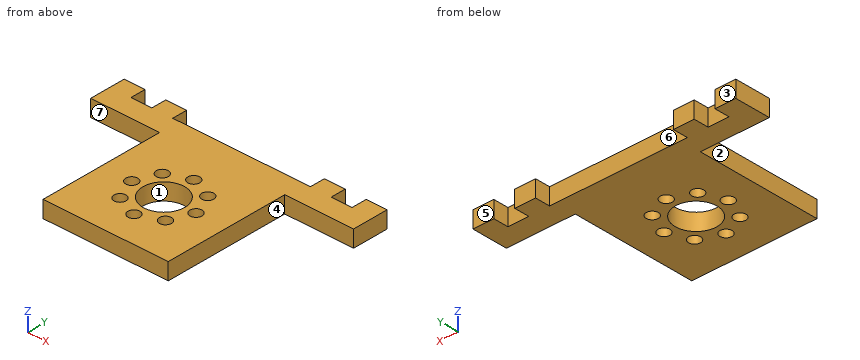
from build123d import *

# Parameters (mm, degrees)
BOSS_EXTRUDE1_DEPTH = 5.08
SKETCH3_W           = 6.35
SKETCH3_H           = 4.572
BOSS_EXTRUDE2_DEPTH = 5.08
SKETCH4_R           = 6.35
SKETCH4_R_2         = 1.8288
CUT_EXTRUDE1_DEPTH  = 5.08
SKETCH5_W           = 29.19984
SKETCH5_H           = 4.572
CUT_EXTRUDE2_DEPTH  = 5.08


with BuildPart() as part:
    # Sketch1 → Boss-Extrude1 (new body)
    with BuildSketch(Plane.XY):
        Polygon((-22.91953125, 7.590234375), (-22.91953125, 1.240234375), (-1.96961125, 1.240234375), (-1.96961125, -36.859765625), (36.13038875, -36.859765625), (36.13038875, 1.240234375), (57.08030875, 1.240234375), (57.08030875, 7.590234375), align=None)
    extrude(amount=BOSS_EXTRUDE1_DEPTH)

    # Sketch3 → Boss-Extrude2 (add)
    with BuildSketch(Plane(origin=(0, 0, 0), x_dir=(-1, 0, 0), z_dir=(0, 0, -1))):
        with Locations((19.74453125, 9.876234375)):
            Rectangle(SKETCH3_W, SKETCH3_H)
        with Locations((7.04453125, 9.876234375)):
            Rectangle(SKETCH3_W, SKETCH3_H)
        with Locations((-5.65546875, 9.876234375)):
            Rectangle(SKETCH3_W, SKETCH3_H)
        with Locations((-28.50530875, 9.876234375)):
            Rectangle(SKETCH3_W, SKETCH3_H)
        with Locations((-41.20530875, 9.876234375)):
            Rectangle(SKETCH3_W, SKETCH3_H)
        with Locations((-53.90530875, 9.876234375)):
            Rectangle(SKETCH3_W, SKETCH3_H)
    extrude(amount=-BOSS_EXTRUDE2_DEPTH)

    # Sketch4 → Cut-Extrude1 (cut)
    with BuildSketch(Plane.XY.offset(5.08)):
        with Locations((17.08038875, -17.809765625)):
            Circle(SKETCH4_R)
        with Locations((7.30138875, -17.809765625)):
            Circle(SKETCH4_R_2)
        with Locations((10.165591537, -10.894968412)):
            Circle(SKETCH4_R_2)
        with Locations((17.08038875, -8.030765625)):
            Circle(SKETCH4_R_2)
        with Locations((23.995185963, -10.894968412)):
            Circle(SKETCH4_R_2)
        with Locations((26.85938875, -17.809765625)):
            Circle(SKETCH4_R_2)
        with Locations((23.995185963, -24.724562838)):
            Circle(SKETCH4_R_2)
        with Locations((17.08038875, -27.588765625)):
            Circle(SKETCH4_R_2)
        with Locations((10.165591537, -24.724562838)):
            Circle(SKETCH4_R_2)
    extrude(amount=-CUT_EXTRUDE1_DEPTH, mode=Mode.SUBTRACT)

    # Sketch5 → Cut-Extrude2 (cut)
    with BuildSketch(Plane.XY.offset(5.08)):
        with Locations((17.08038875, 9.876234375)):
            Rectangle(SKETCH5_W, SKETCH5_H)
    extrude(amount=-CUT_EXTRUDE2_DEPTH, mode=Mode.SUBTRACT)


solid = part.part
Read the model definition and answer for the solid it produces. Units are mm, in the model's axes. Face numbers are marked on the shaded views. A direction names the side the tool comes from. Give positions to 0.01 mm unless a question says otherwise; leave off trailing zeros. Write each loop counter-clockwise with the first axis right and the second up, starting at its lowest first coordinate (ties: lowest second). Pieces come first, ordered by that corner, then holes. Notation, with made-up numbers: (77.5, 85.25) - (126.5, 85.25) arc R26 cw to (126.5, 115.25) - close; hole circle Ø5 at (86, 62). An arc over 180 degrees is marked (long way). Use CSV: the item, a comma, the result in double quotes. Start each with the question number.
(1) Given P1, Ø1.5, axis at x = -7.5, z = 1.5, coming from the -Y side; P2, Ø2, axis at y = -3.5, z = 3.5, coming from the +X side; P3, Ø2.5, axis at x = 48, z = 1.5, coming from the +Y side, each flat-ended and moving along its own axis, determine where each tip first touches the part or whether it passes through.
(2) Find section C-C (z = 1). Count the separate pieces of the cut face and the enclosed holes in it, plus the area to 4 significant figures.
(3) Find section A-A (x = 18). Give the vertices of the cut face in (y, z).
(4) For the marked faces 4, 5, 6 and 7, determine the directions among +Z, -Z, +X, -X, +Y, -Y from which every point of the face is accessible in a straight line to the end or side of a thin tool.
(5) Find section D-D (x = 47). Give the vertices of the cut face in (y, z), plus the area to 3 significant figures.
(6) Find section B-B (y = -22). Give the vertices of the cut face in (x, z).
(7) Consider line 1 along X through (y, z) = (-27.5, 3.9); line 2 along X through (y, z) = (-14, 3.85); line 3 along Y through (x, z) = (-10, 2.1). Determine where each line is inside the solid, lowest interval first.
(8) Determine the mould class of the marked faces 1, 2 and 3 for opening direction Y: +Y half, -Y half, draft (parallel to the pull), parting line (faces both ways), or undercut.
Findings below:
1,P1,"y = 1.24"
1,P2,"x = 36.13"
1,P3,"y = 7.59"
2,separate pieces,"1"
2,enclosed holes,"9"
2,area,"1,865 mm2"
3,outline,"(-36.86, 0) - (-29.17, 0) - (-29.17, 5.08) - (-36.86, 5.08) - close; (-26.01, 0) - (-24.09, 0) - (-24.09, 5.08) - (-26.01, 5.08) - close; (-11.53, 0) - (-9.61, 0) - (-9.61, 5.08) - (-11.53, 5.08) - close; (-6.45, 0) - (7.59, 0) - (7.59, 5.08) - (-6.45, 5.08) - close"
4,face 4,"+Z, -Z, +X, -Y"
4,face 5,"+Z, -Z, +X, -X, +Y"
4,face 6,"+Z, -Z, +Y"
4,face 7,"+Z, -Z, -X, -Y"
5,outline,"(1.24, 0) - (7.59, 0) - (7.59, 5.08) - (1.24, 5.08) - close"
5,area,"32.3 mm2"
6,outline,"(-1.97, 0) - (12.31, 0) - (12.31, 5.08) - (-1.97, 5.08) - close; (21.85, 0) - (36.13, 0) - (36.13, 5.08) - (21.85, 5.08) - close"
7,line 1,"-1.97 to 15.25, 18.91 to 36.13"
7,line 2,"-1.97 to 12, 22.16 to 36.13"
7,line 3,"1.24 to 12.16"
8,face 1,"undercut"
8,face 2,"draft"
8,face 3,"+Y half"
